The model under review builds one solid part; all positions refer to its coordinate system, in mm. Face numbers are marked on the shaded views. A direction names the side the tool comes from. Round coordinates to 2 decimals unless told otherwise and drop trailing zeros. Write each loop counter-clockwise with the first axis right and the second up, starting at its lowest first coordinate (ties: lowest second). Pieces come first, ordered by that corner, then holes. Notation, with made-up numbers: (54, 35.25) -> (85, 35.25) arc R26 cw to (85, 60.25) -> close; hole circle Ø5 at (19, 26.5). An arc over 180 degrees is marked (long way). Answer as a JSON object with one key per item and string values. Group by question number.
1) Insertion check: pin 1 Ø10 at (x, y) = (-18.5, 3) entering from -Z; pin 2 Ø5 at (y, z) = (3.5, -10.5) entering from -X; pin 3 Ø5 at (x, z) = (-18.76, 10.83) entering from +Y; pin 4 Ø9.5 at (x, z) = (21.34, -3.76) entering from +Y. Each pin has a flat end and moves straight along its axis. Give the tip position at first contact, or say it passes through.
2) We need section C-C, the plane z = -18. Write out the cut boundary in (x, y).
3) Machinability: for the marked faces 1, 2 and 3, which of the approach directions +Z, -Z, +X, -X, +Y, -Y give a long, thin tool a straight path to every point of the face, cutting with its end or side? Answer none if there is none.
4) We need section D-D, the plane x = -20. Write out the cut boundary in (y, z).
5) We need section B-B, the plane x = 0. Write out the cut boundary in (y, z).
6) Mouldability with a two-part tool opening along Z and no side actions: class the marked faces 4, 5 and 6 as pulls with the +Z half, pulls with the -Z half, needs draft (parallel to the pull), parting line crosses it, or undercut.
7) We need section A-A, the plane z = 0. Write out the cut boundary in (x, y).
8) To check wall thickness, follow probe 1 along X at (y, z) = (4.5, -19); probe 2 along X at (y, z) = (4.5, -6.5); probe 3 along X at (y, z) = (9.5, 0). State the ranges of each line that lie inside material, in increasing order. Write a range as [from, to].
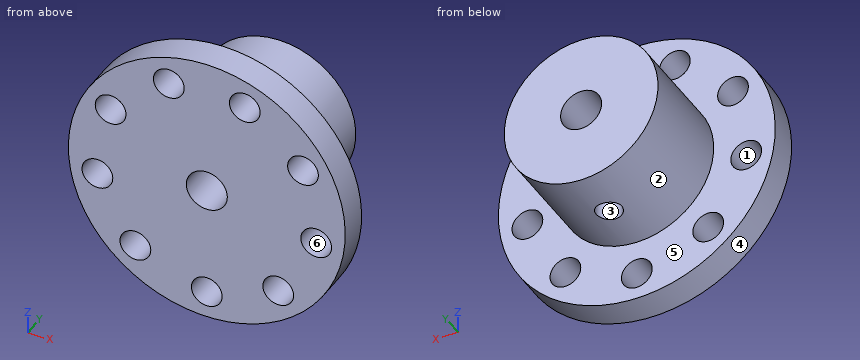
from build123d import *

# Parameters (mm, degrees)
SKETCH_1_R          = 27
SKETCH_1_R_2        = 3
SKETCH_1_R_3        = 4
EXTRUDE_1_DEPTH     = 6
SKETCH_3_R          = 15
SKETCH_3_R_2        = 4
EXTRUDE_2_DEPTH     = 20.4
SKETCH_5_R          = 2.5
CUT_EXTRUDE_1_DEPTH = 47.421546721


with BuildPart() as part:
    # 草图1 → 凸台-拉伸1 (new body)
    with BuildSketch(Plane(origin=(0, 0, 0), x_dir=(1, 0, 0), z_dir=(0, 1, 0))):
        with Locations(Location((0, 0, 0), (0, 0, 270))):
            Circle(SKETCH_1_R)
        with Locations(Location((0, 21.6648374, 0), (0, 0, 270))):
            Circle(SKETCH_1_R_2, mode=Mode.SUBTRACT)
        with Locations(Location((13.925889047, 16.596228301, 0), (0, 0, 270))):
            Circle(SKETCH_1_R_2, mode=Mode.SUBTRACT)
        with Locations(Location((21.335699839, 3.762059534, 0), (0, 0, 270))):
            Circle(SKETCH_1_R_2, mode=Mode.SUBTRACT)
        with Locations(Location((18.762299557, -10.8324187, 0), (0, 0, 270))):
            Circle(SKETCH_1_R_2, mode=Mode.SUBTRACT)
        with Locations(Location((7.409810793, -20.358287835, 0), (0, 0, 270))):
            Circle(SKETCH_1_R_2, mode=Mode.SUBTRACT)
        with Locations(Location((-7.409810793, -20.358287835, 0), (0, 0, 270))):
            Circle(SKETCH_1_R_2, mode=Mode.SUBTRACT)
        with Locations(Location((-18.762299557, -10.8324187, 0), (0, 0, 270))):
            Circle(SKETCH_1_R_2, mode=Mode.SUBTRACT)
        with Locations(Location((-21.335699839, 3.762059534, 0), (0, 0, 270))):
            Circle(SKETCH_1_R_2, mode=Mode.SUBTRACT)
        with Locations(Location((-13.925889047, 16.596228301, 0), (0, 0, 270))):
            Circle(SKETCH_1_R_2, mode=Mode.SUBTRACT)
        with Locations(Location((0, 0, 0), (0, 0, 270))):
            Circle(SKETCH_1_R_3, mode=Mode.SUBTRACT)
    extrude(amount=EXTRUDE_1_DEPTH)

    # 草图3 → 凸台-拉伸2 (add)
    with BuildSketch(Plane(origin=(0, 6, 0), x_dir=(1, 0, 0), z_dir=(0, 1, 0))):
        with Locations(Location((0, 0, 0), (0, 0, 270))):
            Circle(SKETCH_3_R)
        with Locations(Location((0, 0, 0), (0, 0, 270))):
            Circle(SKETCH_3_R_2, mode=Mode.SUBTRACT)
    extrude(amount=EXTRUDE_2_DEPTH)

    # 草图5 → 切除-拉伸1 (cut, through all)
    with BuildSketch(Plane(origin=(0, 0, 0), x_dir=(0, 1, 0), z_dir=(0, 0, 1))):
        with Locations((16.2, 0)):
            Circle(SKETCH_5_R)
    extrude(amount=-CUT_EXTRUDE_1_DEPTH, mode=Mode.SUBTRACT)


solid = part.part
Here are the results:
{
 "1": {"pin 1": "stops at z = -23.38", "pin 2": "stops at x = -25.79", "pin 3": "passes through", "pin 4": "stops at y = 6"},
 "2": {"outline": "(-20.12, 0) -> (-16.58, 0) -> (-16.58, 6) -> (-20.12, 6) -> close; (-11.27, 0) -> (11.27, 0) -> (11.27, 6) -> (-11.27, 6) -> close; (16.58, 0) -> (20.12, 0) -> (20.12, 6) -> (16.58, 6) -> close"},
 "3": {"face 1": "+Y, -Y", "face 2": "+Y", "face 3": "-Z"},
 "4": {"outline": "(0, -18.14) -> (6, -18.14) -> (6, -6.45) -> (0, -6.45) -> close; (0, -1.08) -> (6, -1.08) -> (6, 8.1) -> (0, 8.1) -> close; (0, 13.57) -> (6, 13.57) -> (6, 18.14) -> (0, 18.14) -> close"},
 "5": {"outline": "(0, -27) -> (6, -27) -> (6, -24.66) -> (0, -24.66) -> close; (0, -18.66) -> (6, -18.66) -> (6, -15) -> (13.7, -15) -> (13.7, -4) -> (0, -4) -> close; (0, 4) -> (26.4, 4) -> (26.4, 15) -> (6, 15) -> (6, 27) -> (0, 27) -> close; (18.7, -15) -> (26.4, -15) -> (26.4, -4) -> (18.7, -4) -> close"},
 "6": {"face 4": "parting line crosses it", "face 5": "needs draft", "face 6": "undercut"},
 "7": {"outline": "(-27, 0) -> (-4, 0) -> (-4, 26.4) -> (-15, 26.4) -> (-15, 6) -> (-27, 6) -> close; (4, 0) -> (27, 0) -> (27, 6) -> (15, 6) -> (15, 26.4) -> (4, 26.4) -> close"},
 "8": {"probe 1": "x = [-19.18, -15.72], [-12.13, -1.38], [1.38, 12.13], [15.72, 19.18]", "probe 2": "x = [-26.21, -22.56], [-20.11, 20.11], [22.56, 26.21]", "probe 3": "x = [-15, -4], [4, 15]"}
}
